Source: CAD feature listing. Evaluate the final solid. Frame: model axes, mm. A direction names the side the tool comes from. Give positions to 0.01 mm unless a question says otherwise; leave off trailing zeros. Write each loop counter-clockwise with the first axis right and the second up, starting at its lowest first coordinate (ties: lowest second). Pieces come first, ordered by that corner, then holes.
```python
from build123d import *

# Parameters (mm, degrees)
BOSS_EXTRUDE1_DEPTH     = 6
FILLET1_R               = 0.9525
FILLET2_R               = 2.8575
F_1_4_CLEARANCE_HOLE1_D = 6.7564
CUT_EXTRUDE1_REACH      = 34.312
SKETCH7_R               = 2.5


with BuildPart() as part:
    # Sketch3 → Boss-Extrude1 (new, symmetric)
    with BuildSketch(Plane.XY):
        Polygon((4.7625, 25.4), (0, 25.4), (0, 0), (19.05, 0), (19.05, 4.7625), (4.7625, 4.7625), align=None)
    extrude(amount=BOSS_EXTRUDE1_DEPTH, both=True)

    # Fillet1
    fillet1_edges = [part.edges().sort_by_distance(p)[0] for p in [
        (4.7625, 4.7625, 0),
        (19.05, 4.7625, 0),
        (4.7625, 25.4, 0),
    ]]
    fillet(fillet1_edges, radius=FILLET1_R)

    # Fillet2
    fillet2_edges = [part.edges().sort_by_distance(p)[0] for p in [
        (0, 0, 0),
    ]]
    fillet(fillet2_edges, radius=FILLET2_R)

    # 1/4 Clearance Hole1 (through all)
    with Locations(Plane(origin=(0, 0, 0), x_dir=(-1, 0, 0), z_dir=(0, -1, 0))):
        with Locations((-10.95375, 0)):
            Hole(F_1_4_CLEARANCE_HOLE1_D / 2)

    # Sketch7 → Cut-Extrude1 (cut, up to next)
    with BuildSketch(Plane.ZY, mode=Mode.PRIVATE) as cut_extrude1_sk1:
        with Locations(Location((0, 17.4, 0), (0, 0, 270))):
            Circle(SKETCH7_R)
    cut_extrude1_tool1 = extrude(cut_extrude1_sk1.sketch, amount=-CUT_EXTRUDE1_REACH, mode=Mode.PRIVATE) & part.part
    add(cut_extrude1_tool1.solids().sort_by_distance((0, 17.4, 0))[0], mode=Mode.SUBTRACT)


solid = part.part
```
1. Line query: L1, parallel to Z at x = 2.9, y = 17.4; L2, parallel to Y at x = 9.5, z = 4.25. Output: solid intervals per line, ascending.
2. Mould query, pull axis Z, two halves, no side actions, for faces 1 (the flat face through (3, 7, 6)), 2 (the flat face through (0, 14, 0)), 3 (the cylindrical face through (2.3, 19.4, -1.5)). Classes: +Z half, -Z half, draft (parallel to the pull), parting line (faces both ways), or undercut.
3. Contact query for flat-ended pins moving along their axis: P1, Ø5, axis at x = 10, z = -0.5, coming from the +Y side; P2, Ø6, axis at y = 14, z = 1.5, coming from the +X side. Output: stop coordinate, or through.
4. Cut plane A-A, the plane z = 0. State how many separate pieces and enclosed holes the cut face has, then the cut area to 3 significant figures.
5. Cut plane B-B, the plane y = 17.4. Return the cut outline in (x, z).
6. Cut plane C-C, the plane x = 13.25. Return the cut outline in (y, z), then the cut area to 3 significant figures.
7. Access query for faces 4 (the flat face through (2, 25.4, 0)), 5 (the flat face through (15, 4.762, 0)). Directions: +Z, -Z, +X, -X, +Y, -Y. A direction counts if a zero-diameter tool reaches every point of the face in a straight line with its end or side. Return the directions, or none.
Response values:
1. L1: z = -6 to -2.5, 2.5 to 6
1. L2: y = 0 to 4.76
2. face 1: +Z half
2. face 2: draft
2. face 3: undercut
3. P1: stops at y = 4.76
3. P2: stops at x = 4.76
4. separate pieces: 3
4. enclosed holes: 0
4. area: 131 mm2
5. outline: (0, -6) - (4.76, -6) - (4.76, -2.5) - (0, -2.5) - close; (0, 2.5) - (4.76, 2.5) - (4.76, 6) - (0, 6) - close
6. outline: (0, -6) - (4.76, -6) - (4.76, -2.48) - (0, -2.48) - close; (0, 2.48) - (4.76, 2.48) - (4.76, 6) - (0, 6) - close
6. area: 33.5 mm2
7. face 4: +Z, -Z, +X, -X, +Y
7. face 5: +Z, -Z, +X, +Y
